Source: CAD feature listing. Evaluate the final solid. Frame: model axes, mm. A direction names the side the tool comes from. Coordinates: 2 decimals unless noted, no trailing zeros. Loops run counter-clockwise (first coordinate to the right, second up) from the corner with the lowest first, then second, coordinate; pieces in that order, holes last. Notation, with made-up numbers: M -6.75,-24.75 L 6.25,-24.75 A12 ccw 6.25,-18.75 Z; hole C 12.5,-14 d5. An arc over 180 degrees is marked long. Write each question's results on one line, items separated by ' | '. Start each with the question number.
from build123d import *

# Parameters (mm, degrees)
RECTANGLE027_W   = 20
RECTANGLE027_H   = 650
EXTRUDE063_DEPTH = 20
RECTANGLE026_W   = 200
RECTANGLE026_H   = 800
EXTRUDE062_DEPTH = 20


with BuildPart() as extrude063:
    # Rectangle027 → Extrude063 (new body)
    with BuildSketch(Plane(origin=(289.620605, 275.315636, 420), x_dir=(1, 0, 0), z_dir=(0, 0, 1))):
        with Locations((10, 325)):
            Rectangle(RECTANGLE027_W, RECTANGLE027_H)
    extrude(amount=-EXTRUDE063_DEPTH)


with BuildPart() as extrude063_1:
    # Extrude063 placement: moved
    add(extrude063.part.moved(Location((-149.620605, -150.315636, -100))))


with BuildPart() as cut015:
    # Rectangle026 → Extrude062 (new body)
    with BuildSketch(Plane(origin=(207.600586, 206.495789, 400), x_dir=(1, 0, 0), z_dir=(0, 0, 1))):
        with Locations((100, 400)):
            Rectangle(RECTANGLE026_W, RECTANGLE026_H)
    extrude(amount=EXTRUDE062_DEPTH)


with BuildPart() as cut015_1:
    # Extrude062 placement: moved
    add(cut015.part.moved(Location((-157.600586, -156.495789, -100))))

    # Cut015: cut Extrude063
    add(extrude063_1.part, mode=Mode.SUBTRACT)


solid = cut015_1.part
Item 1: Access query for faces 1 (the flat face through (250, 444, 310)), 2 (the flat face through (150, 125, 310)). Directions: +Z, -Z, +X, -X, +Y, -Y. A direction counts if a zero-diameter tool reaches every point of the face in a straight line with its end or side. Return the directions, or none.
Item 2: Cut plane C-C (y = 430.5). Output: boundary loops of the cut face in (x, z), then the cut area to 3 significant figures.
Item 3: Mould query, pull axis X, two halves, no side actions, for faces 3 (the flat face through (171, 456, 320)), 4 (the flat face through (160, 445, 310)), 5 (the flat face through (150, 775, 310)), 6 (the flat face through (50, 444, 310)). Classes: +X half, -X half, draft (parallel to the pull), parting line (faces both ways), or undercut.
Item 4: Cut plane A-A (x = 152.5). Output: boundary loops of the cut face in (y, z).
Item 5: Line query: probe 1 along X at (y, z) = (284, 306.5); probe 2 along Y at (x, z) = (156, 306.5). Output: solid intervals per line, ascending.
Item 6: Cut plane B-B (z = 308.75). Output: boundary loops of the cut face in (x, y), then the cut area to 3 significant figures.
Response values:
1) face 1: +Z, -Z, +X, +Y, -Y | face 2: +Z, -Z
2) outline: M 50,300 L 140,300 L 140,320 L 50,320 Z; M 160,300 L 250,300 L 250,320 L 160,320 Z | area: 3,600 mm2
3) face 3: draft | face 4: undercut | face 5: undercut | face 6: -X half
4) outline: M 50,300 L 125,300 L 125,320 L 50,320 Z; M 775,300 L 850,300 L 850,320 L 775,320 Z
5) probe 1: x = 50 to 140, 160 to 250 | probe 2: y = 50 to 125, 775 to 850
6) outline: M 50,50 L 250,50 L 250,850 L 50,850 Z; hole M 140,125 L 160,125 L 160,775 L 140,775 Z | area: 147,000 mm2
